```python
from build123d import *

# Parameters (mm, degrees)
EXTRUDE_1_DEPTH = 3


with BuildPart() as part:
    # 草图1 → 凸台-拉伸1 (new body)
    with BuildSketch(Plane.XY):
        with BuildLine():
            ThreePointArc((0, 6), (4.242640687, 4.242640687), (6, 0))
            Line((6, 0), (27, 0))
            ThreePointArc((27, 0), (28.757359313, 4.242640687), (33, 6))
            Line((33, 6), (0, 6))
        make_face()
        with BuildLine():
            Line((27, 0), (6, 0))
            ThreePointArc((6, 0), (4.242640687, -4.242640687), (0, -6))
            Line((0, -6), (33, -6))
            ThreePointArc((33, -6), (28.757359313, -4.242640687), (27, 0))
        make_face()
        with BuildLine():
            ThreePointArc((-2.5, 0), (0, 2.5), (2.5, 0))
            Line((2.5, 0), (6, 0))
            ThreePointArc((6, 0), (4.242640687, 4.242640687), (0, 6))
            ThreePointArc((0, 6), (-4.242640687, 4.242640687), (-6, 0))
            Line((-6, 0), (-2.5, 0))
        make_face()
        with BuildLine():
            Line((6, 0), (2.5, 0))
            ThreePointArc((2.5, 0), (0, -2.5), (-2.5, 0))
            Line((-2.5, 0), (-6, 0))
            ThreePointArc((-6, 0), (-4.242640687, -4.242640687), (0, -6))
            ThreePointArc((0, -6), (4.242640687, -4.242640687), (6, 0))
        make_face()
        with BuildLine():
            ThreePointArc((33, 6), (28.757359313, 4.242640687), (27, 0))
            Line((27, 0), (30.5, 0))
            ThreePointArc((30.5, 0), (33, 2.5), (35.5, 0))
            Line((35.5, 0), (39, 0))
            ThreePointArc((39, 0), (37.242640687, 4.242640687), (33, 6))
        make_face()
        with BuildLine():
            Line((30.5, 0), (27, 0))
            ThreePointArc((27, 0), (28.757359313, -4.242640687), (33, -6))
            ThreePointArc((33, -6), (37.242640687, -4.242640687), (39, 0))
            Line((39, 0), (35.5, 0))
            ThreePointArc((35.5, 0), (33, -2.5), (30.5, 0))
        make_face()
    extrude(amount=EXTRUDE_1_DEPTH)


solid = part.part
```
Can you work these out from the model? Positions are in its coordinate system, mm. Give positions to 0.01 mm unless a question says otherwise; leave off trailing zeros. Loops run counter-clockwise (first coordinate to the right, second up) from the corner with the lowest first, then second, coordinate; pieces in that order, holes last. Notation, with made-up numbers: M 20,-7.5 L 34,-7.5 A15 ccw 34,12.5 Z; hole C 34,86 d1. An arc over 180 degrees is marked long. Use one line per item in the form item = value. Start each with the question number.
(1) I want a section at A-A, the plane z = 1.75. Write out the boundary of the cut face in (x, y), and give its area (3 significant figures).
(2) I want a section at B-B, the plane x = -1. Write out the boundary of the cut face in (y, z).
(3) I want a section at D-D, the plane y = 4.75. Write out the boundary of the cut face in (x, z).
(4) Please list where these lines run through material, in increasing order: line 1 (Y direction, x = 0, z = 1.05); line 2 (X direction, y = 2, z = 2.2); line 3 (X direction, y = 0.75, z = 0.75).
(5) I'm going to push a flat-ended pin straight in: P1, Ø1.5, axis at y = 4.5, z = 2, coming from the -X side. Where does the tip first touch, or does it pass through?
(6) Thinking about a two-plate mould opening in X: for faces 1 (the cylindrical face through (35.31, 0.96, 1.48)), 2 (the flat face through (16, 0, 0)), which applies, released by +X, released by -X, zero draft, split by the parting line, or undercut?
(7) I want a section at C-C, the plane y = 1.5. Write out the boundary of the cut face in (x, z), and give its area (3 significant figures).
Worked out:
q1.outline = M 0,-6 L 33,-6 A6 ccw 33,6 L 0,6 A6 ccw Z; hole C 0,0 d5; hole C 33,0 d5
q1.area = 470 mm²
q2.outline = M -5.92,0 L -2.29,0 L -2.29,3 L -5.92,3 Z; M 2.29,0 L 5.92,0 L 5.92,3 L 2.29,3 Z
q3.outline = M -3.67,0 L 36.67,0 L 36.67,3 L -3.67,3 Z
q4.line_1 = -6 to -2.5, 2.5 to 6
q4.line_2 = -5.66 to -1.5, 1.5 to 31.5, 34.5 to 38.66
q4.line_3 = -5.95 to -2.38, 2.38 to 30.62, 35.38 to 38.95
q5.P1 = -4.68
q6.face_1 = undercut
q6.face_2 = zero draft
q7.outline = M -5.81,0 L -2,0 L -2,3 L -5.81,3 Z; M 2,0 L 31,0 L 31,3 L 2,3 Z; M 35,0 L 38.81,0 L 38.81,3 L 35,3 Z
q7.area = 110 mm²
